from build123d import *

# Parameters (mm, degrees)
PAD_DEPTH             = 10
POCKET_DEPTH          = 10
SKETCH009_W           = 3.913781
SKETCH009_H           = 10.54203
POCKET001_DEPTH       = 2
POLARPATTERN002_COUNT = 2
CHAMFER_SIZE          = 0.6
SKETCH011_W           = 0.658057
SKETCH011_H           = 11.036716
POCKET002_DEPTH       = 5
BODY_PLACEMENT_ANGLE  = 90


with BuildPart() as part:
    # Sketch001 → Pad (new body, symmetric)
    with BuildSketch(Plane.XZ):
        Polygon((-8.4, 0), (-8.4, -5.15), (8.4, -5.15), (8.4, -2.15), (2.5, -2.15), (2.5, 0), (2.5, 1.8), (-2.5, 1.8), (-2.5, 0), align=None)
    extrude(amount=PAD_DEPTH, both=True)

    # Sketch → Pocket (cut, symmetric)
    with BuildSketch(Plane.XY):
        with BuildLine():
            ThreePointArc((-2.2, 1.187434), (-2.5, 0), (-2.2, -1.187434))
            Line((-2.2, -1.187434), (-2.2, -5.5))
            Line((-2.2, -5.5), (4.8, -5.5))
            Line((4.722171, -2.539952), (4.8, -5.5))
            ThreePointArc((4.722171, -2.539952), (4.263597, -2.023905), (3.771176, -2.507761))
            Line((4.3, -4.344865), (3.771176, -2.507761))
            Line((3.244578, -4.864673), (4.3, -4.344865))
            Line((1.6, -4.864673), (3.244578, -4.864673))
            Line((1.6, -3.743474), (1.6, -4.864673))
            Line((2.677439, -3.432031), (1.6, -3.743474))
            Line((2.2, -1.187434), (2.677439, -3.432031))
            ThreePointArc((2.2, -1.187434), (2.5, 0), (2.2, 1.187434))
            Line((2.2, 1.187434), (2.677439, 3.432031))
            Line((2.677439, 3.432031), (1.6, 3.743474))
            Line((1.6, 3.743474), (1.6, 4.864673))
            Line((1.6, 4.864673), (3.244578, 4.864673))
            Line((3.244578, 4.864673), (4.3, 4.344865))
            Line((4.3, 4.344865), (3.650118, 2.519747))
            ThreePointArc((3.650118, 2.519747), (4.169872, 1.907371), (4.829785, 2.365262))
            Line((4.829785, 2.365262), (4.8, 5.5))
            Line((-2.2, 5.5), (4.8, 5.5))
            Line((-2.2, 1.187434), (-2.2, 5.5))
        make_face()
    extrude(amount=POCKET_DEPTH, both=True, mode=Mode.SUBTRACT)

    # Sketch009 → Pocket001 (cut, symmetric)
    with BuildSketch(Plane.XY):
        with Locations((3.133439, 0)):
            Rectangle(SKETCH009_W, SKETCH009_H)
    extrude(amount=POCKET001_DEPTH, both=True, mode=Mode.SUBTRACT)

    # Sphere001 → Sphere001 (revolve, cut)
    with BuildSketch(Plane(origin=(5, 0, -5.15), x_dir=(1, 0, 0), z_dir=(0, 1, 0))):
        with BuildLine():
            ThreePointArc((0, -1), (1, 0), (0, 1))
            Line((0, 1), (0, -1))
        make_face()
    sphere001 = revolve(axis=Axis((5, 0, -5.15), (0, 0, -1)), mode=Mode.SUBTRACT)

    # PolarPattern002: Sphere001 ×2 about axis
    polarpattern002_axis = Axis((0, 0, 0), (0, 0, 1))
    for i in range(1, POLARPATTERN002_COUNT):
        add(sphere001.rotate(polarpattern002_axis, i * 360 / POLARPATTERN002_COUNT), mode=Mode.SUBTRACT)

    # Chamfer
    chamfer_edges = [part.edges().sort_by_distance(p)[0] for p in [
        (8.4, 0, -5.15),
        (0, -10, -5.15),
        (0, 10, -5.15),
        (-8.4, 0, -5.15),
        (8.4, -10, -3.65),
        (8.4, 10, -3.65),
        (-8.4, -10, -2.575),
        (-8.4, 10, -2.575),
    ]]
    chamfer(chamfer_edges, length=CHAMFER_SIZE)

    # Sketch011 → Pocket002 (cut)
    with BuildSketch(Plane.XY):
        with Locations((-2.269595, 0)):
            Rectangle(SKETCH011_W, SKETCH011_H)
    extrude(amount=POCKET002_DEPTH, mode=Mode.SUBTRACT)


with BuildPart() as part_1:
    # Body placement: moved
    add(part.part.moved(Location((0, 0, -10))).rotate(Axis((0, 0, -10), (0, 0, -1)), BODY_PLACEMENT_ANGLE))


solid = part_1.part
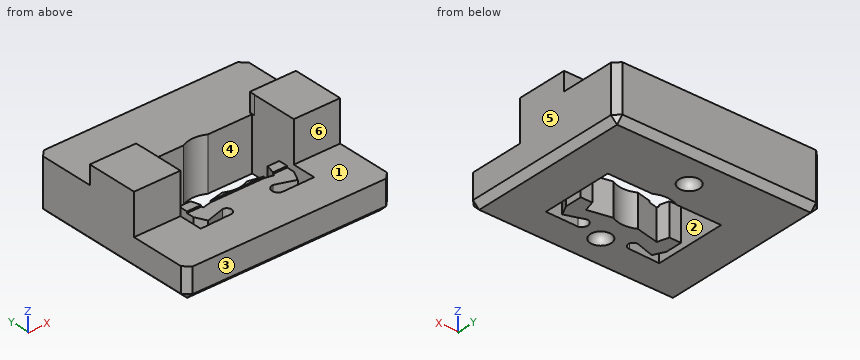
For this review, take the finished solid that the model builds, in its own axes (mm). Face numbers are marked on the shaded views. A direction names the side the tool comes from. Round coordinates to 2 decimals unless told otherwise and drop trailing zeros. Write each loop counter-clockwise with the first axis right and the second up, starting at its lowest first coordinate (ties: lowest second). Pieces come first, ordered by that corner, then holes. Notation, with made-up numbers: M 47.25,42.25 L 51.25,42.25 A14 cw 51.25,68.25 Z; hole C 25,-12.75 d7. An arc over 180 degrees is marked long. Write item = value, one per line. Start each with the question number.
(1) For line 1 along X through (y, z) = (-3.5, -13); line 2 along X through (y, z) = (0.75, -11.75); line 3 along Y through (x, z) = (-1.5, -10.5), list the stretches that pass through material, from the lowest coordinate up.
(2) Clearance check with flat-ended pins moving along their axes: pin 1 Ø0.5 at (x, y) = (4.5, -2) entering from +Z; pin 2 Ø3 at (x, z) = (-2, -10) entering from -Y; pin 3 Ø3 at (x, y) = (5, 4.5) entering from +Z. State where each tip first meets the part, or that it passes through.
(3) We need section B-B (x = 7). Give the boundary of the cut face in (y, z), then the cut area to 3 significant figures.
(4) The part is to be moulded in two halves that separate along X. For the marked faces 4, 5 and 6, say which applies: +X half, -X half, draft (parallel to the pull), parting line (faces both ways), or undercut.
(5) For the marked faces 1, 2 and 3, list the 3-axis set-ups (+Z, -Z, +X, -X, +Y, -Y) from which the entire face can be reached by the end or side of a thin tool; tool diameter is ignored.
(6) We need section C-C (y = -3). Give the boundary of the cut face in (x, z).
(7) We need section D-D (z = -10.5). Give the boundary of the cut face in (x, y).
Results found:
q1.line_1 = -10 to -5.5, -4.74 to 4.74, 5.5 to 10
q1.line_2 = -10 to -5.5, 5.5 to 10
q1.line_3 = 2.2 to 8.4
q2.pin_1 = -12
q2.pin_2 = 2.2
q2.pin_3 = -10
q3.outline = M -8.4,-14.55 L -7.8,-15.15 L 7.8,-15.15 L 8.4,-14.55 L 8.4,-10 L 2.5,-10 L 2.5,-8.2 L -2.5,-8.2 L -2.5,-12.15 L -8.4,-12.15 Z
q3.area = 82.5 mm²
q4.face_4 = undercut
q4.face_5 = +X half
q4.face_6 = draft
q5.face_1 = +Z, +X, -X, -Y
q5.face_2 = +Z, -Z
q5.face_3 = +Z, -Z, +X, -X, -Y
q6.outline = M -10,-14.55 L -9.4,-15.15 L -5.5,-15.15 L -5.5,-12.15 L -10,-12.15 Z; M -4.86,-15.15 L 4.86,-15.15 L 4.86,-12.15 L -4.86,-12.15 Z; M 5.5,-15.15 L 9.4,-15.15 L 10,-14.55 L 10,-12.15 L 5.5,-12.15 Z
q7.outline = M -10,-2.5 L -5.5,-2.5 L -5.5,2.2 L -1.19,2.2 A2.5 cw 1.19,2.2 L 5.5,2.2 L 5.5,-2.5 L 10,-2.5 L 10,7.8 L 9.4,8.4 L -9.4,8.4 L -10,7.8 Z
